```python
from build123d import *

# Parameters (mm, degrees)
SKETCH1_W           = 15.039204539
SKETCH1_H           = 10.543027195
SKETCH1_W_2         = 15.2
SKETCH1_H_2         = 2
BOSS_EXTRUDE1_DEPTH = 4.9


with BuildPart() as part:
    # Sketch1 → Boss-Extrude1 (new body)
    with BuildSketch(Plane(origin=(0, 0, 0), x_dir=(1, 0, 0), z_dir=(0, 1, 0))):
        Polygon((2.4, 0), (17.6, 0), (17.6, -2), (20, -2), (20, 0), (20, 18), (0, 18), (0, 0), (0, -2), (2.4, -2), align=None)
        with Locations((9.91960227, 7.744546306)):
            Rectangle(SKETCH1_W, SKETCH1_H, mode=Mode.SUBTRACT)
        with Locations((10, 15.5)):
            Rectangle(SKETCH1_W_2, SKETCH1_H_2, mode=Mode.SUBTRACT)
    extrude(amount=BOSS_EXTRUDE1_DEPTH)


solid = part.part
```
For this review, take the finished solid that the model builds, in its own axes (mm). A direction names the side the tool comes from. Round coordinates to 2 decimals unless told otherwise and drop trailing zeros. Loops run counter-clockwise (first coordinate to the right, second up) from the corner with the lowest first, then second, coordinate; pieces in that order, holes last.
Q1. Add section A-A on z = 0.25. Write out the cut boundary in (x, y).
Result sheet:
outline: (0, 0) - (2.4, 0) - (2.4, 4.9) - (0, 4.9) - close; (17.6, 0) - (20, 0) - (20, 4.9) - (17.6, 4.9) - close
Q2. Add section C-C on x = 7.75. Write out the cut boundary in (y, z), plus the area to 3 significant figures.
Result sheet:
outline: (0, -18) - (4.9, -18) - (4.9, -16.5) - (0, -16.5) - close; (0, -14.5) - (4.9, -14.5) - (4.9, -13.02) - (0, -13.02) - close; (0, -2.47) - (4.9, -2.47) - (4.9, 0) - (0, 0) - close
area: 26.7 mm2
Q3. To check wall thickness, follow line 1 along Z through (x, y) = (5.5, 4.3); line 2 along X through (y, z) = (1.95, -9); line 3 along X through (y, z) = (1.35, 0.25). State the ranges of each line that lie inside material, in increasing order.
Result sheet:
line 1: z = -18 to -16.5, -14.5 to -13.02, -2.47 to 0
line 2: x = 0 to 2.4, 17.44 to 20
line 3: x = 0 to 2.4, 17.6 to 20
Q4. Add section B-B on y = 2.35. Write out the cut boundary in (x, z).
Result sheet:
outline: (0, -18) - (20, -18) - (20, 2) - (17.6, 2) - (17.6, 0) - (2.4, 0) - (2.4, 2) - (0, 2) - close; hole (2.4, -16.5) - (17.6, -16.5) - (17.6, -14.5) - (2.4, -14.5) - close; hole (2.4, -13.02) - (17.44, -13.02) - (17.44, -2.47) - (2.4, -2.47) - close
Q5. Mouldability with a two-part tool opening along X and no side actions: class faces 4 (the face through (10, 0, -1)), 5 (the face through (17.6, 2, -15)), 6 (the face through (20, 2, -8)) as +X half, -X half, draft (parallel to the pull), parting line (faces both ways), or undercut.
Result sheet:
face 4: draft
face 5: undercut
face 6: +X half
Q6. Insertion check: pin 1 Ø2.5 at (x, y) = (9, 2) entering from +Z. The pin has a flat end and moves straight along its axis. Give the tip position at first contact, or say it passes through.
Result sheet:
pin 1: stops at z = 0
Q7. Machinability: for faces 1 (the face through (10, 2, -14.5)), 2 (the face through (1, 2, 2)), 3 (the face through (10, 2, 0)), which of the approach directions +Z, -Z, +X, -X, +Y, -Y give a long, thin tool a straight path to every point of the face, cutting with its end or side? Answer none if there is none.
Result sheet:
face 1: +Y, -Y
face 2: +Z, +X, -X, +Y, -Y
face 3: +Z, +Y, -Y
Q8. Add section D-D on z = -7.25. Write out the cut boundary in (x, y).
Result sheet:
outline: (0, 0) - (2.4, 0) - (2.4, 4.9) - (0, 4.9) - close; (17.44, 0) - (20, 0) - (20, 4.9) - (17.44, 4.9) - close
